The model under review builds one solid part; all positions refer to its coordinate system, in mm. Face numbers are marked on the shaded views. A direction names the side the tool comes from. Round coordinates to 2 decimals unless told otherwise and drop trailing zeros. Order: outer loops, then holes, each group sorted by start corner. A loop starts at its lowest first (then second) coordinate and runs counter-clockwise, first axis right, second up.
1) Clearance check with flat-ended pins moving along their axes: P1, Ø4, axis at y = 10.5, z = -73, coming from the -X side; P2, Ø1, axis at x = -20.5, z = -21.5, coming from the -Y side; P3, Ø1, axis at x = -12.5, y = 9.5, coming from the +Z side; P4, Ø10, axis at y = 6, z = -12.5, coming from the -X side. State where each tip first meets the part, or that it passes through.
2) To check wall thickness, follow L1, parallel to X at y = 6.25, z = -80; L2, parallel to Z at x = -125, y = 5.75; L3, parallel to X at y = 14, z = 0. State the ranges of each line that lie inside material, in increasing order.
3) Machinability: for the marked faces 1 and 2, which of the approach directions +Z, -Z, +X, -X, +Y, -Y give a long, thin tool a straight path to every point of the face, cutting with its end or side? Answer none if there is none.
4) Consider section A-A (z = -80). Give the boundary of the cut face in (x, y).
5) Mouldability with a two-part tool opening along X and no side actions: class the marked faces 3, 4, 5 and 6 as pulls with the +X half, pulls with the -X half, needs draft (parallel to the pull), parting line crosses it, or undercut.
6) Consider section D-D (x = -94). Give the boundary of the cut face in (y, z), then the cut area to 3 significant figures.
7) Consider section B-B (y = 11). Give the boundary of the cut face in (x, z), then the cut area to 3 significant figures.
8) Consider section C-C (x = -5). Give the boundary of the cut face in (y, z), then the cut area to 3 significant figures.
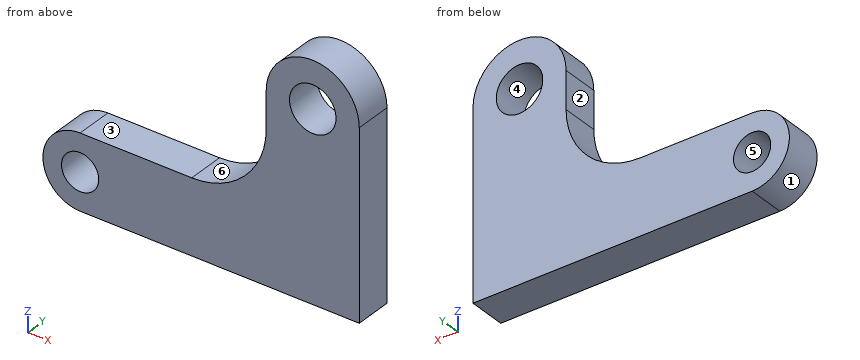
Autodesk Fusion 360 part; units mm, degrees
sketch "Sketch1" plane through (0, 0, 0) normal (0, 1, 0) x (1, 0, 0)
  line L0 (24.3392, -13.8982) -> (-125.6608, -13.8982)
  arc A0 (-125.6608, -13.8982) -> (-125.6608, -53.8982) centre (-125.6608, -33.8982) ccw
  arc A1 (-14.3201, -29.8888) -> (-14.3202, -29.8887) centre (-14.3202, -29.8888) ccw
  line L1 (-14.3201, -29.8888) -> (-14.3201, -30.0005)
  arc A2 (-25.6608, -113.8982) -> (24.3392, -113.8982) centre (-0.6608, -113.8982) ccw
  line L2 (24.3392, -113.8982) -> (24.3392, -13.8982)
  line L3 (-125.6608, -53.8982) -> (-65.6608, -53.8982)
  arc A3 (-25.6608, -93.8982) -> (-65.6608, -53.8982) centre (-65.6608, -93.8982) ccw
  line L4 (-25.6608, -93.8982) -> (-25.6608, -113.8982)
  circle A4 centre (-0.6608, -113.8982) radius 12.5
  circle A5 centre (-125.6608, -33.8982) radius 10
  dimension "d1" = 100
  dimension "d2" = 150
  dimension "d3" = 20
  dimension "d4" = 25
  dimension "d5" = 40
  dimension "d6" = 25
  dimension "d7" = 20
sketch "Sketch2" plane through (0, 0, 0) normal (0, 1, 0) x (1, 0, 0)
  line L0 (25, 100) -> (-125, 100)
  arc A0 (-125, 100) -> (-125, 60) centre (-125, 80) ccw
  line L1 (-125, 60) -> (-25, 60)
  line L2 (-25, 60) -> (-25, 0)
  arc A1 (-25, 0) -> (25, 0) centre (0, 0) ccw
  line L3 (25, 0) -> (25, 100)
  circle A2 centre (0, 0) radius 12.5
  circle A3 centre (-125, 80) radius 10
  dimension "d10" = 150
  dimension "d11" = 100
  dimension "d12" = 25
  dimension "d13" = 20
  dimension "d14" = 25
  dimension "d15" = 20
extrude "Extrude2" add sketch "Sketch2" along normal blind 20
fillet "Fillet1" radius 40 1 edges at (-25, 10, -60)
Answer below:
1. P1: stops at x = -144.36
1. P2: stops at y = 0
1. P3: stops at z = 21.93
1. P4: stops at x = -25
2. L1: x = -145 to -135, -115 to 25
2. L2: z = -100 to -90, -70 to -60
2. L3: x = -25 to -12.5, 12.5 to 25
3. face 1: -X, +Y, -Y
3. face 2: +Z, -X, +Y, -Y
4. outline: (-145, 0) - (-135, 0) - (-135, 20) - (-145, 20) - close; (-115, 0) - (25, 0) - (25, 20) - (-115, 20) - close
5. face 3: needs draft
5. face 4: undercut
5. face 5: undercut
5. face 6: pulls with the -X half
6. outline: (0, -100) - (20, -100) - (20, -60) - (0, -60) - close
6. area: 800 mm2
7. outline: (-125, -100) - (25, -100) - (25, 0) arc R25 ccw to (-25, 0) - (-25, -20) arc R40 cw to (-65, -60) - (-125, -60) arc R20 ccw to start; hole circle Ø20 at (-125, -80); hole circle Ø25 at (0, 0)
7. area: 10,100 mm2
8. outline: (0, -100) - (20, -100) - (20, -11.46) - (0, -11.46) - close; (0, 11.46) - (20, 11.46) - (20, 24.49) - (0, 24.49) - close
8. area: 2,030 mm2
